from build123d import *

# Parameters (mm, degrees)
CHANFRO1_SIZE = 2
FILETE1_R     = 5


with BuildPart() as part:
    # Esboço1 → Revolução1 (revolve)
    with BuildSketch(Plane(origin=(0, 0, 0), x_dir=(0, 0, -1), z_dir=(1, 0, 0))):
        with BuildLine():
            Line((100, 0), (100, 15))
            Line((100, 15), (70, 15))
            Line((70, 15), (70, 22.5))
            Line((70, 22.5), (60, 22.5))
            Line((60, 22.5), (60, 35))
            Line((60, 35), (6.614378278, 35))
            ThreePointArc((6.614378278, 35), (0, 32.5), (-6.614378278, 35))
            Line((-6.614378278, 35), (-60, 35))
            Line((-60, 35), (-60, 22.5))
            Line((-60, 22.5), (-70, 22.5))
            Line((-70, 22.5), (-70, 15))
            Line((-70, 15), (-100, 15))
            Line((-100, 15), (-100, 0))
            Line((-100, 0), (100, 0))
        make_face()
    revolve(axis=Axis((0, 0, 100), (0, 0, -1)))

    # Chanfro1
    chanfro1_edges = [part.edges().sort_by_distance(p)[0] for p in [
        (0, -15, 100),
        (0, -15, -100),
    ]]
    chamfer(chanfro1_edges, length=CHANFRO1_SIZE)

    # Filete1
    filete1_edges = [part.edges().sort_by_distance(p)[0] for p in [
        (0, -15, 70),
        (0, -22.5, 60),
        (0, -22.5, -60),
        (0, -15, -70),
    ]]
    fillet(filete1_edges, radius=FILETE1_R)


solid = part.part
Here's how the part is built. I have some questions about the finished solid (model axes, mm). A direction names the side the tool comes from. Round coordinates to 2 decimals unless told otherwise and drop trailing zeros. Order: outer loops, then holes, each group sorted by start corner. A loop starts at its lowest first (then second) coordinate and runs counter-clockwise, first axis right, second up. Notation, with made-up numbers: (-29, 66) -> (3, 66) arc R16 ccw to (3, 81) -> close; hole circle Ø9 at (34.5, -28.5). An arc over 180 degrees is marked (long way). Return JSON: item names as keys, results as strings.
Q1. I need wall thicknesses on line 1 along Z through (x, y) = (-13.5, -14); line 2 along X through (y, z) = (-1, -80); line 3 along X through (y, z) = (1, 66.5). Which ranges of each line are inside material? Lowest first, please. Write a range as from..to.
Filled sheet:
{"line 1": "z = -70.03..70.03", "line 2": "x = -14.97..14.97", "line 3": "x = -22.48..22.48"}
Q2. For pin 1 Ø1 at (x, z) = (-4, 47) entering from +Y; pin 2 Ø4 at (x, z) = (3.5, -11) entering from -Y; pin 3 Ø1.5 at (x, y) = (-20.5, -22.5) entering from +Z, each with a flat end and sliding along its axis, tell me the tip position at first contact or that it passes through.
Filled sheet:
{"pin 1": "stops at y = 34.82", "pin 2": "stops at y = -34.97", "pin 3": "stops at z = 60"}
Q3. If we section it at B-B on z = 83: List the corners of the cut face in (x, y) for me, plus the area to 3 significant figures.
Filled sheet:
{"outline": "circle Ø30 at (0, 0)", "area": "707 mm^2"}
Q4. Which directions (+Z, -Z, +X, -X, +Y, -Y) give clear straight access to the entire face, cutting with the end or side of a thin tool? Please do faces 1 (the cylindrical face through (-19.961, 10.382, -67.465)), 2 (the flat face through (0, 0, 100)), 3 (the flat face through (-1.6, -20.1, 70)).
Filled sheet:
{"face 1": "-Z", "face 2": "+Z, +X, -X, +Y, -Y", "face 3": "+Z"}
Q5. If we section it at A-A on z = 0: List the corners of the cut face in (x, y) for me, plus the area to 3 significant figures.
Filled sheet:
{"outline": "circle Ø65 at (0, 0)", "area": "3,320 mm^2"}
